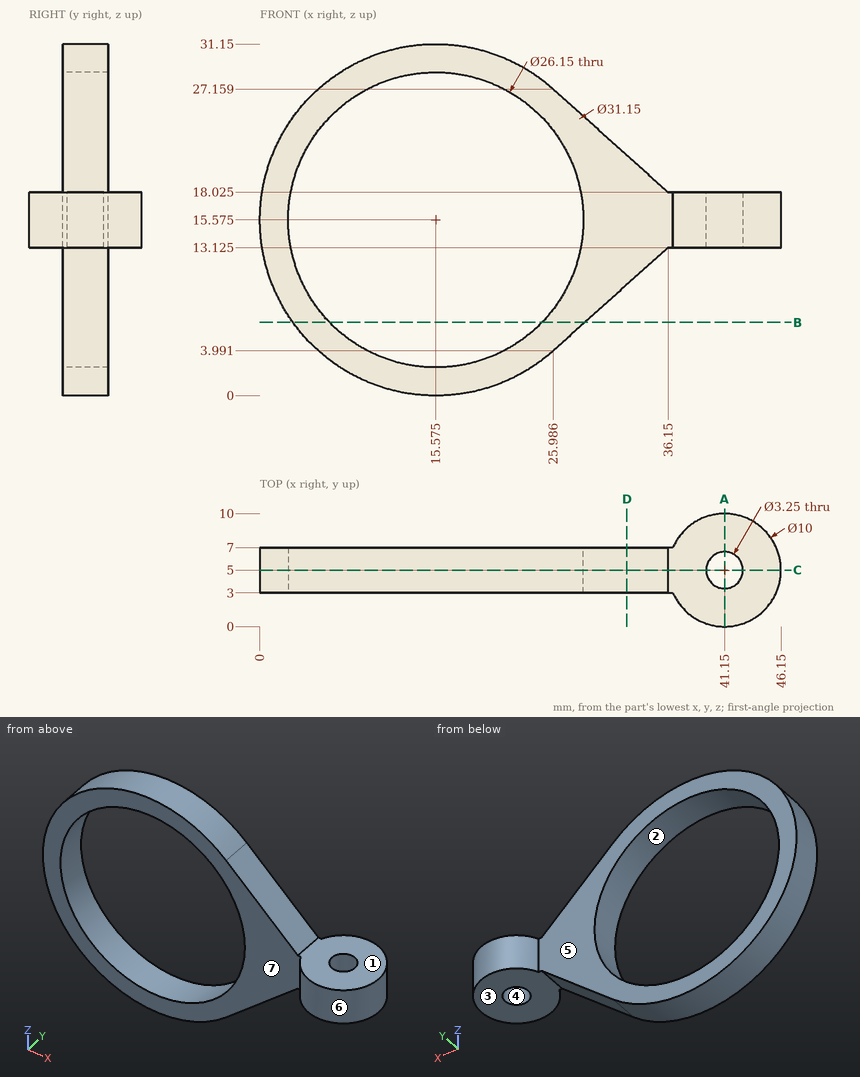
Study the drawing (mm; zero at the part's minimum x, y, z) and answer. A direction names the side the tool comes from. Round coordinates to 2 decimals unless told otherwise and drop trailing zeros. Write each loop counter-clockwise with the first axis right and the second up, starting at its lowest first coordinate (ties: lowest second). Pieces come first, ordered by that corner, then holes.
1) Given pin 1 Ø10 at (x, z) = (25.5, 4) entering from -Y; pin 2 Ø5 at (x, y) = (21.5, 2.5) entering from +Z; pin 3 Ø3.5 at (x, y) = (41.15, 5) entering from -Z (3 decimals), each flat-ended and moving along its own axis, determine where each tip first touches the part or whether it passes through.
2) A cutting plane is placed at B-B (z = 6.5). Give the vertices of the cut face in (x, y).
3) A cutting plane is placed at A-A (x = 41.15). Give the vertices of the cut face in (y, z) (1 decimal).
4) The mould has two halves that part along Z. Classify the marked faces 1, 2, 3 and 4: pulls with the +Z half, pulls with the -Z half, needs draft (parallel to the pull), parting line crosses it, or undercut.
5) A cutting plane is placed at D-D (x = 32.5). Give the vertices of the cut face in (y, z) (1 decimal).
6) A tool of negligible diameter and unlimited length cuts with its end or side. For the marked faces 5, 6 and 7, from which of +Z, -Z, +X, -X, +Y, -Y can it reach the whole face along a straight path? Write none if from no direction.
7) A cutting plane is placed at C-C (y = 5). Give the number of separate pieces and of enclosed holes in the cut face, plus the area to 3 significant figures.
8) Straight lines are drawn through the part: line 1 (Y direction, x = 9, z = 3.5); line 2 (Z direction, x = 19, y = 6); line 3 (X direction, y = 3.75, z = 6). For each, find the intervals that lie inside material, in ascending order.
Completed:
1. pin 1: stops at y = 3
1. pin 2: stops at z = 30.76
1. pin 3: stops at z = 13.125
2. outline: (2.92, 3) - (6.16, 3) - (6.16, 7) - (2.92, 7) - close; (24.99, 3) - (28.78, 3) - (28.78, 7) - (24.99, 7) - close
3. outline: (0, 13.1) - (3.4, 13.1) - (3.4, 18) - (0, 18) - close; (6.6, 13.1) - (10, 13.1) - (10, 18) - (6.6, 18) - close
4. face 1: pulls with the +Z half
4. face 2: undercut
4. face 3: pulls with the -Z half
4. face 4: needs draft
5. outline: (3, 9.8) - (7, 9.8) - (7, 21.3) - (3, 21.3) - close
6. face 5: +Z, -Z, -X, +Y
6. face 6: +Z, -Z
6. face 7: +Z, -Z, -X, -Y
7. separate pieces: 2
7. enclosed holes: 1
7. area: 318 mm2
8. line 1: y = 3 to 7
8. line 2: z = 0.38 to 2.96, 28.19 to 30.77
8. line 3: x = 3.29 to 6.67, 24.48 to 28.22
